```python
from build123d import *

# Parameters (mm, degrees)
EXTRUDE_1_DEPTH          = 5
CUT_EXTRUDE_1_DEPTH      = 19.708286934
CUT_EXTRUDE_1_DEPTH_BACK = 19.708286934
SKETCH_2_R               = 1.5


with BuildPart() as part:
    # 草图1 → 凸台-拉伸1 (new body)
    with BuildSketch(Plane.XY):
        with BuildLine():
            Line((-5, 5), (-5, 0.5))
            ThreePointArc((-5, 0.5), (-5.146446609, 0.146446609), (-5.5, 0))
            Line((-5.5, 0), (-15, 0))
            Line((-15, 0), (-15, 1))
            Line((-15, 1), (-6.5, 1))
            ThreePointArc((-6.5, 1), (-6.146446609, 1.146446609), (-6, 1.5))
            Line((-6, 1.5), (-6, 5))
            ThreePointArc((-6, 5), (0, 11), (6, 5))
            Line((6, 5), (6, 1.5))
            ThreePointArc((6, 1.5), (6.146446609, 1.146446609), (6.5, 1))
            Line((6.5, 1), (15, 1))
            Line((15, 1), (15, 0))
            Line((15, 0), (5.5, 0))
            ThreePointArc((5.5, 0), (5.146446609, 0.146446609), (5, 0.5))
            Line((5, 0.5), (5, 5))
            ThreePointArc((5, 5), (0, 10), (-5, 5))
        make_face()
    extrude(amount=EXTRUDE_1_DEPTH)

    # 草图2 → 切除-拉伸1 (cut, two sides: drawn at the far end of the back side and taken through both)
    with BuildSketch(Plane(origin=(0, 1, 0), x_dir=(1, 0, 0), z_dir=(0, 1, 0)).offset(-CUT_EXTRUDE_1_DEPTH_BACK)):
        with Locations(Location((-10, -2.5, 0), (0, 0, 270))):
            Circle(SKETCH_2_R)
        with Locations(Location((10, -2.5, 0), (0, 0, 270))):
            Circle(SKETCH_2_R)
    extrude(amount=CUT_EXTRUDE_1_DEPTH + CUT_EXTRUDE_1_DEPTH_BACK, mode=Mode.SUBTRACT)


solid = part.part
```
Source: CAD feature listing. Evaluate the final solid. Frame: model axes, mm. A direction names the side the tool comes from. Coordinates: 2 decimals unless noted, no trailing zeros. Order: outer loops, then holes, each group sorted by start corner. A loop starts at its lowest first (then second) coordinate and runs counter-clockwise, first axis right, second up. Notation, with made-up numbers: M 9,-26.5 L 58,-26.5 A35 ccw 58,10.5 Z; hole C 46.25,69 d11. An arc over 180 degrees is marked long. Write each question's results on one line, items separated by ' | '. Start each with the question number.
1) Draft query along X for faces 1 (the face through (-5, 3, 2)), 2 (the face through (15, 0.5, 2.5)), 3 (the face through (-15, 0.5, 2.5)). Return one class per face: released by +X, released by -X, zero draft, split by the parting line, or undercut.
2) Section query D-D (x = 2.75). Return the cut outline in (y, z).
3) Section query A-A (x = -10). Return the cut outline in (y, z), plus the area to 3 significant figures.
4) Section query B-B (z = 2.5). Return the cut outline in (x, y).
5) Access query for faces 4 (the face through (-6, 3, 2)), 5 (the face through (6, 3, 2)), 6 (the face through (5, 3, 2)). Directions: +Z, -Z, +X, -X, +Y, -Y. A direction counts if a zero-diameter tool reaches every point of the face in a straight line with its end or side. Return the directions, or none.
6) Line query: line 1 (X direction, y = 0.75, z = 2.5); line 2 (Z direction, x = 10, y = 0.3); line 3 (X direction, y = 2.25, z = 3.35). Output: solid intervals per line, ascending. Write a range as from..to.
7) Section query C-C (y = 3). Return the cut outline in (x, z), plus the area to 3 significant figures.
8) Contact query for flat-ended pins moving along their axis: pin 1 Ø1.8 at (y, z) = (2.5, 1.5) entering from +X; pin 2 Ø2.5 at (x, z) = (10, 2.5) entering from -Y; pin 3 Ø2 at (y, z) = (3.5, 3) entering from -X; pin 4 Ø1.5 at (x, z) = (-12, 3) entering from +Y. Output: stop coordinate, or through.
Answers:
1) face 1: undercut | face 2: released by +X | face 3: released by -X
2) outline: M 9.18,0 L 10.33,0 L 10.33,5 L 9.18,5 Z
3) outline: M 0,0 L 1,0 L 1,1 L 0,1 Z; M 0,4 L 1,4 L 1,5 L 0,5 Z | area: 2.00 mm^2
4) outline: M -15,0 L -11.5,0 L -11.5,1 L -15,1 Z; M -8.5,0 L -5.5,0 A0.5 ccw -5,0.5 L -5,5 A5 cw 5,5 L 5,0.5 A0.5 ccw 5.5,0 L 8.5,0 L 8.5,1 L 6.5,1 A0.5 cw 6,1.5 L 6,5 A6 ccw -6,5 L -6,1.5 A0.5 cw -6.5,1 L -8.5,1 Z; M 11.5,0 L 15,0 L 15,1 L 11.5,1 Z
5) face 4: +Z, -Z, -X, +Y | face 5: +Z, -Z, +X, +Y | face 6: +Z, -Z, -Y
6) line 1: x = -15..-11.5, -8.5..-5, 5..8.5, 11.5..15 | line 2: z = 0..1, 4..5 | line 3: x = -6..-5, 5..6
7) outline: M -6,0 L -5,0 L -5,5 L -6,5 Z; M 5,0 L 6,0 L 6,5 L 5,5 Z | area: 10.0 mm^2
8) pin 1: stops at x = 6 | pin 2: passes through | pin 3: stops at x = -6 | pin 4: stops at y = 1
